```python
from build123d import *

# Parameters (mm, degrees)
F0_R     = 1.6
F1_DEPTH = 1.5


with BuildPart() as f1:
    # F0 (on Front) → F1 (new body)
    with BuildSketch(Plane.XZ):
        with BuildLine():
            ThreePointArc((33.895837, 22.340272), (28.643297, 32.919956), (16.970563, 31.112698))
            Line((16.970563, 31.112698), (13.096545, 27.662792))
            ThreePointArc((13.096545, 27.662792), (0.969919, 22.633346), (-11.662681, 26.206554))
            Line((-11.662681, 26.206554), (-17.246483, 31.378249))
            ThreePointArc((-17.246483, 31.378249), (-29.552007, 32.386435), (-33.457384, 20.673605))
            ThreePointArc((-33.457384, 20.673605), (-33.705418, 18.848308), (-35.340534, 18))
            Line((-35.340534, 18), (-36.4, 18))
            ThreePointArc((-36.4, 18), (-39.228427, 16.828427), (-40.4, 14))
            Line((-40.4, 14), (-40.4, 0))
            Line((-40.4, 0), (-40.4, -14))
            ThreePointArc((-40.4, -14), (-39.228427, -16.828427), (-36.4, -18))
            Line((-36.4, -18), (-35.340534, -18))
            ThreePointArc((-35.340534, -18), (-33.705418, -18.848308), (-33.457384, -20.673605))
            ThreePointArc((-33.457384, -20.673605), (-29.552007, -32.386435), (-17.246483, -31.378249))
            Line((-17.246483, -31.378249), (-11.662681, -26.206554))
            ThreePointArc((-11.662681, -26.206554), (0.969919, -22.633346), (13.096545, -27.662792))
            Line((13.096545, -27.662792), (16.970563, -31.112698))
            ThreePointArc((16.970563, -31.112698), (28.643297, -32.919956), (33.895837, -22.340272))
            ThreePointArc((33.895837, -22.340272), (34.336883, -20.711696), (35.866678, -20))
            Line((35.866678, -20), (40, -20))
            ThreePointArc((40, -20), (50.606602, -15.606602), (55, -5))
            Line((55, -5), (55, 0))
            Line((55, 0), (55, 5))
            ThreePointArc((55, 5), (50.606602, 15.606602), (40, 20))
            Line((40, 20), (35.866678, 20))
            ThreePointArc((35.866678, 20), (34.336883, 20.711696), (33.895837, 22.340272))
        make_face()
        with BuildLine():
            ThreePointArc((-34.7, -9.6), (-33.65, -10.65), (-34.7, -11.7))
            Line((-34.7, -11.7), (-36.3, -11.7))
            ThreePointArc((-36.3, -11.7), (-37.35, -10.65), (-36.3, -9.6))
            Line((-36.3, -9.6), (-36.3, -7.8))
            ThreePointArc((-36.3, -7.8), (-37.35, -6.75), (-36.3, -5.7))
            Line((-36.3, -5.7), (-34.7, -5.7))
            ThreePointArc((-34.7, -5.7), (-33.65, -6.75), (-34.7, -7.8))
            Line((-34.7, -7.8), (-34.7, -9.6))
        make_face(mode=Mode.SUBTRACT)
        with Locations((-28.7, -5.7)):
            Circle(F0_R, mode=Mode.SUBTRACT)
        with BuildLine():
            Line((30, -13.9), (32, -13.9))
            ThreePointArc((32, -13.9), (32.8, -14.7), (32, -15.5))
            Line((32, -15.5), (30, -15.5))
            ThreePointArc((30, -15.5), (29.2, -14.7), (30, -13.9))
        make_face(mode=Mode.SUBTRACT)
        with Locations((42, -14)):
            Circle(F0_R, mode=Mode.SUBTRACT)
        with Locations((-28.7, 5.7)):
            Circle(F0_R, mode=Mode.SUBTRACT)
        with BuildLine():
            ThreePointArc((-34.7, 7.8), (-33.65, 6.75), (-34.7, 5.7))
            Line((-34.7, 5.7), (-36.3, 5.7))
            ThreePointArc((-36.3, 5.7), (-37.35, 6.75), (-36.3, 7.8))
            Line((-36.3, 7.8), (-36.3, 9.6))
            ThreePointArc((-36.3, 9.6), (-37.35, 10.65), (-36.3, 11.7))
            Line((-36.3, 11.7), (-34.7, 11.7))
            ThreePointArc((-34.7, 11.7), (-33.65, 10.65), (-34.7, 9.6))
            Line((-34.7, 9.6), (-34.7, 7.8))
        make_face(mode=Mode.SUBTRACT)
        with Locations((15.25, 15.25)):
            Circle(F0_R, mode=Mode.SUBTRACT)
        with BuildLine():
            ThreePointArc((30, 13.9), (29.2, 14.7), (30, 15.5))
            Line((30, 15.5), (32, 15.5))
            ThreePointArc((32, 15.5), (32.8, 14.7), (32, 13.9))
            Line((32, 13.9), (30, 13.9))
        make_face(mode=Mode.SUBTRACT)
        with BuildLine():
            Line((28, -4.5), (28, 0))
            Line((28, 0), (28, 4.5))
            ThreePointArc((28, 4.5), (29.464466, 8.035534), (33, 9.5))
            Line((33, 9.5), (42, 9.5))
            ThreePointArc((42, 9.5), (45.535534, 8.035534), (47, 4.5))
            Line((47, 4.5), (47, 0))
            Line((47, 0), (47, -4.5))
            ThreePointArc((47, -4.5), (45.535534, -8.035534), (42, -9.5))
            Line((42, -9.5), (33, -9.5))
            ThreePointArc((33, -9.5), (29.464466, -8.035534), (28, -4.5))
        make_face(mode=Mode.SUBTRACT)
        with Locations((42, 14)):
            Circle(F0_R, mode=Mode.SUBTRACT)
    extrude(amount=F1_DEPTH)


solid = f1.part
```
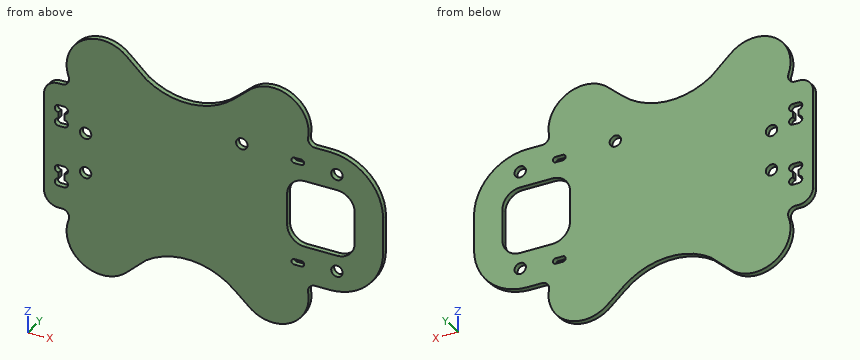
Verification items for the finished model (mm, model axes). Coordinates: 2 decimals unless noted, no trailing zeros. Loops run counter-clockwise (first coordinate to the right, second up) from the corner with the lowest first, then second, coordinate; pieces in that order, holes last. Notation, with made-up numbers: (65, -9) - (71, -9) arc R14 ccw to (71, 8) - close; hole circle Ø3 at (17, 17). An arc over 180 degrees is marked (long way). Return JSON: item names as keys, results as strings.
1. Go/stop test with flat-tipped pins: pin 1 (0.8 mm diameter, centred on x = -35.5, y = -1, fed in from -Z); pin 2 (0.8 mm diameter, centred on x = 31, y = -1, fed in from +Z). Record where each tip stops, or that it passes through.
Established:
{"pin 1": "stops at z = -18.01", "pin 2": "stops at z = 31.59"}
2. Section check C-C, the plane x = 1. Record the boundary of the cut face in (y, z).
Established:
{"outline": "(-1.5, -22.64) - (0, -22.64) - (0, 22.64) - (-1.5, 22.64) - close"}
3. Thickness scan on L1, parallel to Z at x = 42, y = -0.5; L2, parallel to Z at x = 30.5, y = -0.95; L3, parallel to X at y = -1.15, z = -1.5. Record the ranges inside material, lowest first.
Established:
{"L1": "z = -19.87 to -15.6, -12.4 to -9.5, 9.5 to 12.4, 15.6 to 19.87", "L2": "z = -31.68 to -15.5, -13.9 to -8.83, 8.83 to 13.9, 15.5 to 31.68", "L3": "x = -40.4 to 28, 47 to 55"}
4. Section check B-B, the plane y = -1.05. Count the separate pieces of the cut face and the enclosed holes in it, then the cut area to 3 significant figures.
Established:
{"separate pieces": "1", "enclosed holes": "10", "area": "4,470 mm2"}
5. Section check A-A, the plane x = 15.25. Record the boundary of the cut face in (y, z).
Established:
{"outline": "(-1.5, -29.58) - (0, -29.58) - (0, 13.65) - (-1.5, 13.65) - close; (-1.5, 16.85) - (0, 16.85) - (0, 29.58) - (-1.5, 29.58) - close"}
